Autodesk Inventor part; units mm, degrees
ref_plane "YZ Plane" through (0, 0, 0) normal (1, 0, 0) x (0, 1, 0)
ref_plane "XZ Plane" through (0, 0, 0) normal (0, 1, 0) x (-1, 0, 0)
ref_plane "XY Plane" through (0, 0, 0) normal (0, 0, 1) x (1, 0, 0)
sketch "スケッチ1" plane through (0, 0, 0) normal (0, 1, 0) x (-1, 0, 0)
  line L0 (101.7324, -28.9004) -> (451.7324, -28.9004)
  line L1 (451.7324, -28.9004) -> (451.7324, 67.6956)
  arc A0 (451.7324, 67.6956) -> (328.1926, 37.3714) centre (451.7324, -199.1148) ccw
  arc A1 (101.7324, -28.9004) -> (328.1926, 37.3714) centre (48.6916, 572.4068) ccw
  dimension "d1" = 350
  dimension "d2" = 603.642
extrude "押し出し1" add sketch "スケッチ1" along normal blind 70
sketch "スケッチ2" plane through (-101.7324, 0, -28.9004) normal (0, 0, -1) x (-1, 0, 0)
  arc A0 (68.7528, 0) -> (350, 70) centre (68.7528, 600) ccw
  line L0 (350, 0) -> (0, 0)
  line L1 (350, 0) -> (350, 70)
  line L2 (0, 0) -> (0, 70)
  point P0 (-101.7324, 0)
  dimension "d9" = 600
extrude "押し出し2" cut sketch "スケッチ2" against normal through all
shell "シェル1" thickness 2 removed faces 4 at (-334.0598, 39.1147, 40.3449) at (-359.2071, 70, 10.3289) at (-150.6861, 46.6667, -22.5561) at (-325.356, 65.1801, -28.9004)
properties part number "splitter"
Can you work these out from the model? Positions are in its coordinate system, mm. A direction names the side the tool comes from. Round coordinates to 2 decimals unless told otherwise and drop trailing zeros. Loops run counter-clockwise (first coordinate to the right, second up) from the corner with the lowest first, then second, coordinate; pieces in that order, holes last.
Item 1: Suppose I cut it at B-B, the plane z = -7.5. Write out the boundary of the cut face in (x, y).
Item 2: Suppose I cut it at A-A, the plane y = 36. Write out the boundary of the cut face in (x, z), then the cut area to 3 significant figures.
Item 3: Will these pins go through, and if not, where does the flat tip stop? pin 1 Ø5 at (x, z) = (-146.5, -24.5) entering from +Y; pin 2 Ø3 at (x, z) = (-363, 4) entering from +Y; pin 3 Ø12 at (x, y) = (-347, 31) entering from +Z.
Item 4: Please list where these lines run through material, in increasing order: L1, parallel to Y at x = -263, z = -22; L2, parallel to X at y = 61.5, z = 59; L3, parallel to Y at x = -259, z = -7.5.
Item 5: Which directions (+Z, -Z, +X, -X, +Y, -Y) give clear straight access to the entire face, cutting with the end or side of a thin tool? Please do faces 1 (the cylindrical face through (-344.77, 25.87, 7.99)), 2 (the flat face through (-151, 2, -26)).
Reported:
1. outline: (-451.73, 70) arc R600 ccw to (-216.3, 1.75) - (-216.3, 3.76) arc R598 cw to (-447.44, 70) - close
2. outline: (-375.19, -28.9) - (-369.25, -28.9) - (-369.25, 54.63) arc R266.81 ccw to (-375.19, 56.48) - close
2. area: 502 mm2
3. pin 1: stops at y = 2
3. pin 2: stops at y = 34.35
3. pin 3: stops at z = 48.75
4. L1: y = 7.18 to 9.2
4. L2: x = -435.09 to -430.53
4. L3: y = 6.56 to 8.59
5. face 1: +Z, -Z, -X, -Y
5. face 2: +Z, -Z, +X, +Y
